For this review, use the dimensioned drawing (mm, ordinates from the lowest corner) and the shaded views. Give positions to 0.01 mm unless a question says otherwise; leave off trailing zeros. Write each loop counter-clockwise with the first axis right and the second up, starting at its lowest first coordinate (ties: lowest second). Pieces come first, ordered by that corner, then holes.
1) For P1, Ø5.5, axis at x = 198, y = 5.5, coming from the -Z side, flat-tipped, find the tip position at first contact; note if it passes through.
2) Draft analysis for pull direction X (two halves, no side actions). For the marked faces 1 and 2, state which applies: pulls with the +X half, pulls with the -X half, needs draft (parallel to the pull), parting line crosses it, or undercut.
3) Wall thickness on line 1 along X through (y, z) = (2.75, 96); line 2 along Z through (x, y) = (255.5, 1); line 3 along X through (y, z) = (9, 23.5): over which ranges is each line inside the solid? List them lowest first.
4) We need section B-B on z = 117. Give the boundary of the cut face in (x, y).
5) We need section A-A on x = 199. Give the boundary of the cut face in (y, z), and give its area (3 significant figures).
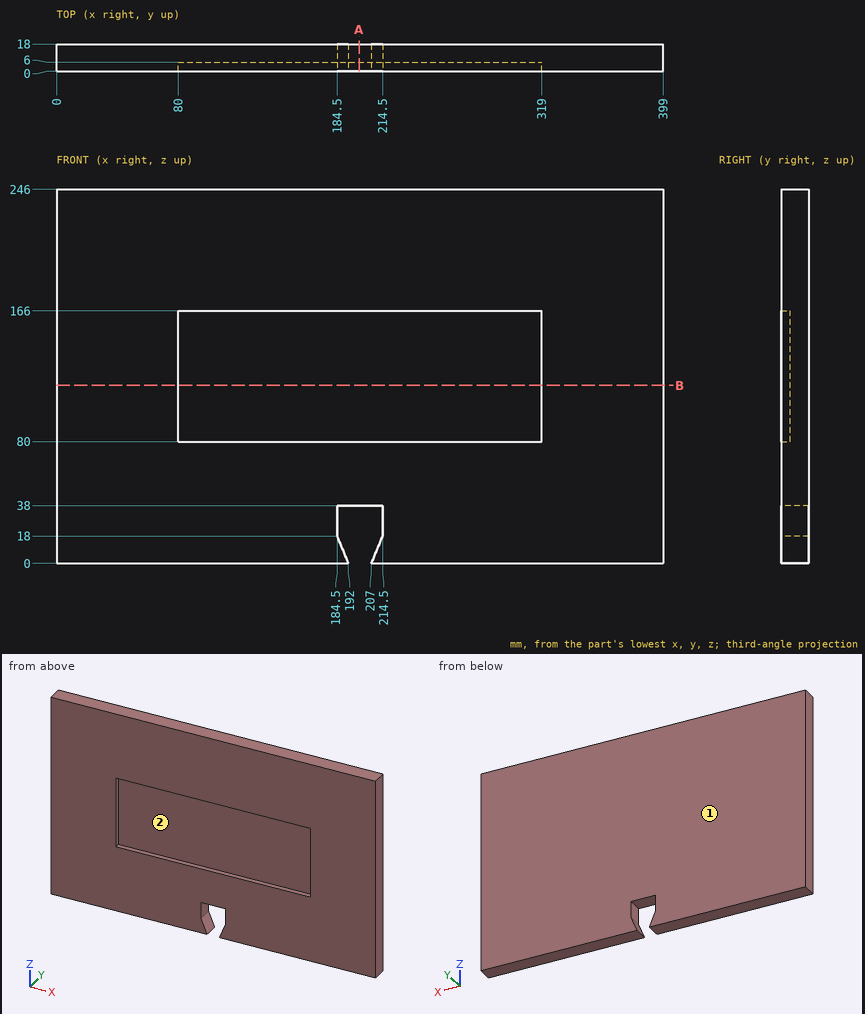
Results list:
1. P1: stops at z = 38
2. face 1: needs draft
2. face 2: undercut
3. line 1: x = 0 to 80, 319 to 399
3. line 2: z = 0 to 80, 166 to 246
3. line 3: x = 0 to 184.5, 214.5 to 399
4. outline: (0, 0) - (80, 0) - (80, 6) - (319, 6) - (319, 0) - (399, 0) - (399, 18) - (0, 18) - close
5. outline: (0, 38) - (18, 38) - (18, 246) - (0, 246) - (0, 166) - (6, 166) - (6, 80) - (0, 80) - close
5. area: 3,230 mm2
